Autodesk Inventor part; units mm, degrees
ref_plane "YZ Plane" through (0, 0, 0) normal (1, 0, 0) x (0, 1, 0)
ref_plane "XZ Plane" through (0, 0, 0) normal (0, 1, 0) x (-1, 0, 0)
ref_plane "XY Plane" through (0, 0, 0) normal (0, 0, 1) x (1, 0, 0)
sketch "Sketch1" plane through (0, 0, 0) normal (0, 0, 1) x (1, 0, 0)
  line L0 (0, 0) -> (-25.4, 0)
  line L1 (-25.4, 0) -> (-25.4, 150)
  line L2 (-25.4, 150) -> (0, 150)
  line L3 (0, 150) -> (0, 0)
  dimension "d0" = 25.4
  dimension "d1" = 150
extrude "Extrusion1" add sketch "Sketch1" along normal blind 5
sketch "Sketch2" plane through (0, 0, 0) normal (0, 0, -1) x (-1, 0, 0)
  point P0 (0, 0)
sketch "Sketch3" plane through (0, 0, 0) normal (0, 0, -1) x (-1, 0, 0)
  line L0 (4.1948, 7.7945) -> (22.3514, 7.7945)
  line L1 (22.3514, 7.7945) -> (22.3514, 7.4454)
  line L2 (22.3514, 7.4454) -> (4.1948, 7.4454)
  line L3 (4.1948, 7.4454) -> (4.1948, 7.7945)
  point P0 (0, 0)
extrude "Extrusion2" add sketch "Sketch3" along normal blind 10
sketch "Sketch4" plane through (-22.3514, 7.4454, 0) normal (0, -1, 0) x (1, 0, 0)
  circle A0 centre (9.6514, -4.8899) radius 4.6183
  point P0 (22.3514, 0)
extrude "Extrusion3" add sketch "Sketch4" along normal blind 20
fillet "Fillet1" radius 2 1 edges at (-17.3183, -12.5546, -4.8899)
sketch "Sketch5" plane through (-12.7, -12.5546, -4.8899) normal (0, -1, 0) x (1, 0, 0)
  circle A0 centre (0, 0) radius 2.6183
  circle A1 centre (0, 0) radius 0.7983
  point P0 (12.7, 4.8899)
extrude "Extrusion4" cut sketch "Sketch5" against normal blind 20 contours A1
sketch "Sketch6" plane through (0, 0, 5) normal (0, 0, 1) x (1, 0, 0)
  circle A0 centre (-13.1019, 144.2767) radius 1
  point P0 (0, 0)
  dimension "d11" = 2
extrude "Extrusion5" cut sketch "Sketch6" against normal blind 20
sketch "Sketch7" plane through (-22.3514, 7.7945, 0) normal (0, 1, 0) x (1, 0, 0)
  circle A0 centre (9.6514, 4.8899) radius 0.7983
  circle A1 centre (9.6514, 4.8899) radius 2.5276
  point P0 (22.3514, 0)
extrude "Extrusion6" add sketch "Sketch7" along normal blind 120
properties part number "spray"
The model under review builds one solid part; all positions refer to its coordinate system, in mm. A direction names the side the tool comes from. Round coordinates to 2 decimals unless told otherwise and drop trailing zeros. Write each loop counter-clockwise with the first axis right and the second up, starting at its lowest first coordinate (ties: lowest second). Pieces come first, ordered by that corner, then holes. Notation, with made-up numbers: (-11.5, -36.75) - (18.5, -36.75) arc R21 cw to (18.5, -25.75) - close; hole circle Ø4 at (-31.75, 34). An arc over 180 degrees is marked (long way). Answer as CSV lines item,"result". Start each with the question number.
(1) To check wall thickness, follow line 1 (Z direction, x = -12.5, y = 42); line 2 (Z direction, x = -12.7, y = -7.5); line 3 (Z direction, x = -3, y = 124). State the ranges of each line that lie inside material, in increasing order.
(2) We need section A-A on y = 31. State the section outline as (x, z) points.
(3) Draft analysis for pull direction Z (two halves, no side actions). For faces 6 (the flat face through (-13, 76, 5)), 7 (the flat face through (-12, -12.555, -4)), 8 (the cylindrical face through (-13.248, 66.954, -7.357)), 9 (the cylindrical face through (-16.365, -1.429, -2.08)), state which applies: pulls with the +Z half, pulls with the -Z half, needs draft (parallel to the pull), parting line crosses it, or undercut.
(4) For faces 1 (the flat face through (-25.4, 74, 2)), 2 (the flat face through (-15.2, 7.794, -3.8)), 3 (the flat face through (-13, 150, 2)), 4 (the flat face through (-13, 0, 2)), 5 (the flat face through (-12.7, 127.794, -3.8)), list the 3-axis set-ups (+Z, -Z, +X, -X, +Y, -Y) from which the entire face can be reached by the end or side of a thin tool; tool diameter is ignored.
(5) For pin 1 Ø2 at (y, z) = (62.5, -6) entering from +X; pin 2 Ø1.5 at (x, z) = (-11.5, 1.5) entering from -Y; pin 3 Ø6 at (x, y) = (-19.5, 99) entering from -Z, all flat-tipped, find the tip position at first contact; note any pin that passes through.
Worked answers:
1,line 1,"-7.41 to -5.66, -4.12 to -2.37, 0 to 5"
1,line 2,"-9.51 to -5.69, -4.09 to -0.27"
1,line 3,"0 to 5"
2,outline,"(-25.4, 0) - (0, 0) - (0, 5) - (-25.4, 5) - close; circle Ø5.06 at (-12.7, -4.89); hole circle Ø1.6 at (-12.7, -4.89)"
3,face 6,"pulls with the +Z half"
3,face 7,"needs draft"
3,face 8,"undercut"
3,face 9,"undercut"
4,face 1,"+Z, -Z, -X, +Y, -Y"
4,face 2,"+Y"
4,face 3,"+Z, -Z, +X, -X, +Y"
4,face 4,"+Z, +X, -X, -Y"
4,face 5,"-Z, +X, -X, +Y"
5,pin 1,"x = -10.17"
5,pin 2,"y = 0"
5,pin 3,"z = 0"
